Autodesk Inventor part; units mm, degrees
ref_plane "YZ Plane" through (0, 0, 0) normal (1, 0, 0) x (0, 1, 0)
ref_plane "XZ Plane" through (0, 0, 0) normal (0, 1, 0) x (-1, 0, 0)
ref_plane "XY Plane" through (0, 0, 0) normal (0, 0, 1) x (1, 0, 0)
sketch "Szkic1" plane through (0, 0, 0) normal (0, 0, 1) x (1, 0, 0)
  circle A0 centre (0, 0) radius 15
  dimension "d0" = 30
extrude "Wyciągnięcie proste1" add sketch "Szkic1" along normal blind 35 and the other way blind 37.5
sketch "Szkic3" plane through (0, 0, 35) normal (0, 0, 1) x (1, 0, 0)
  circle A0 centre (0, 0) radius 10
  circle A1 centre (0, 0) radius 15
  dimension "d4" = 20
  dimension "d5" = 30
extrude "Wyciągnięcie proste2" cut sketch "Szkic3" against normal blind 30
chamfer "Faza1" distance 3.5 angle 45 1 edges at (-15, 0, 5)
sketch "Szkic4" plane through (0, 0, -37.5) normal (0, 0, -1) x (-1, 0, 0)
  circle A0 centre (0, 0) radius 7.5
  circle A1 centre (0, 0) radius 15
  dimension "d11" = 15
  dimension "d12" = 30
extrude "Wyciągnięcie proste3" cut sketch "Szkic4" against normal blind 30
sketch "Szkic8" plane through (0, 0, 35) normal (0, 0, 1) x (1, 0, 0)
  circle A0 centre (0, 0) radius 10
  dimension "d33" = 20
extrude "Wyciągnięcie proste7" add sketch "Szkic8" along normal blind 6
sketch "Szkic9" plane through (0, 0, 41) normal (0, 0, 1) x (1, 0, 0)
  circle A0 centre (0, 0) radius 5.05
  dimension "d36" = 10.1
extrude "Wyciągnięcie proste8" cut sketch "Szkic9" against normal blind 5.5
sketch "Szkic10" plane through (0, 0, 0) normal (1, 0, 0) x (0, 1, 0)
  circle A0 centre (0, 38.5) radius 1.5
  line L0 (-5.05, 41) -> (5.05, 41)
  point P0 (0, 0)
  dimension "d39" = 3
  dimension "d42" = 2.5
extrude "Wyciągnięcie proste9" cut sketch "Szkic10" against normal blind 25
thread "Gwint4"
sketch "Szkic11" plane through (0, 0, 0) normal (1, 0, 0) x (0, 1, 0)
  circle A0 centre (0, -22.5) radius 1.5
  point P0 (0, 0)
  dimension "d45" = 3
extrude "Wyciągnięcie proste10" cut sketch "Szkic11" against normal blind 20
thread "Gwint5"
properties part number "koncowka" material "Aluminium 6061"
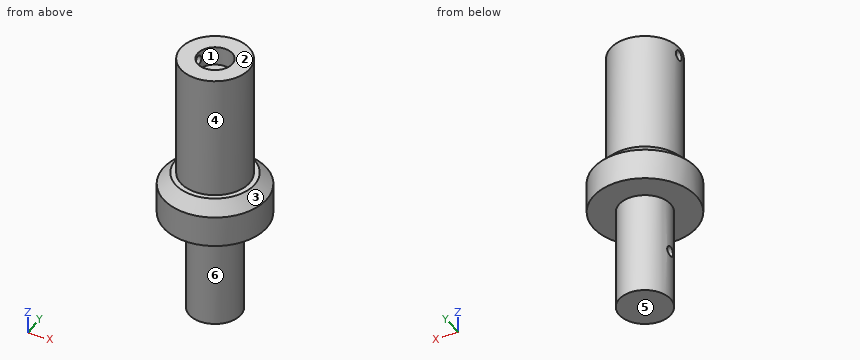
Can you work these out from the model? Positions are in its coordinate system, mm. Face numbers are marked on the shaded views. A direction names the side the tool comes from. Coordinates: 2 decimals unless noted, no trailing zeros. Write each loop counter-clockwise with the first axis right and the second up, starting at its lowest first coordinate (ties: lowest second). Pieces come first, ordered by that corner, then holes. Notation, with made-up numbers: (29, 68.5) - (56, 68.5) arc R36 ccw to (56, 105.5) - close; hole circle Ø7 at (17, 50.5). An arc over 180 degrees is marked (long way). Return JSON: item names as keys, results as strings.
Q1. I'm going to push flat-ended pins straight in: pin 1 Ø6 at (x, z) = (7, -13.5) entering from -Y; pin 2 Ø1.8 at (y, z) = (0, -22.5) entering from -X; pin 3 Ø8 at (x, z) = (-7, -16.5) entering from +Y. Where does each tip first touch, or does it pass through?
Computed values:
{"pin 1": "stops at y = -6.34", "pin 2": "stops at x = 0", "pin 3": "stops at y = 6.87"}
Q2. If we section it at B-B (z = 8): Please give me the cut outline in (x, y), then the cut area to 3 significant figures.
Computed values:
{"outline": "circle Ø20 at (0, 0)", "area": "314 mm2"}
Q3. Please list where these lines run through material, in increasing order: L1, parallel to Z at x = -4.25, y = 0; L2, parallel to Z at x = -5, y = -6; L3, parallel to Y at x = -8.7, z = 38.5. Write a range as from..to.
Computed values:
{"L1": "z = -37.5..-24, -21..35.5", "L2": "z = -7.5..41", "L3": "y = -4.93..-1.5, 1.5..4.93"}
Q4. On a 3-axis mill with a long thin cutter (end or side, diameter ignored), from which of +Z, -Z, +X, -X, +Y, -Y can I reach the whole of each face in a straight line? I mean the marked faces 4, 5 and 6. Say none if no direction works.
Computed values:
{"face 4": "+Z", "face 5": "-Z, +X, -X, +Y, -Y", "face 6": "-Z"}
Q5. If we section it at D-D (z = 38.5): Please give me the cut outline in (x, y), then the cut area to 3 significant figures.
Computed values:
{"outline": "(-9.89, -1.5) arc R10 ccw (long way) to (-9.89, 1.5) - (-4.82, 1.5) arc R5.05 cw (long way) to (-4.82, -1.5) - close", "area": "219 mm2"}
Q6. If we section it at A-A (y = 0): Please give me the cut outline in (x, z).
Computed values:
{"outline": "(-15, -7.5) - (-7.5, -7.5) - (-7.5, -21) - (0, -21) - (0, -24) - (-7.5, -24) - (-7.5, -37.5) - (7.5, -37.5) - (7.5, -7.5) - (15, -7.5) - (15, 1.5) - (11.5, 5) - (10, 5) - (10, 41) - (5.05, 41) - (5.05, 35.5) - (-5.05, 35.5) - (-5.05, 37) - (-10, 37) - (-10, 5) - (-11.5, 5) - (-15, 1.5) - close; (-10, 40) - (-5.05, 40) - (-5.05, 41) - (-10, 41) - close"}
Q7. Thinking about a two-plate mould opening in X: for the marked faces 1, 2 and 3, which applies, +X half, -X half, draft (parallel to the pull), parting line (faces both ways), or undercut?
Computed values:
{"face 1": "undercut", "face 2": "draft", "face 3": "parting line"}
Q8. If we section it at C-C (z = 0): Please give me the cut outline in (x, y).
Computed values:
{"outline": "circle Ø30 at (0, 0)"}
